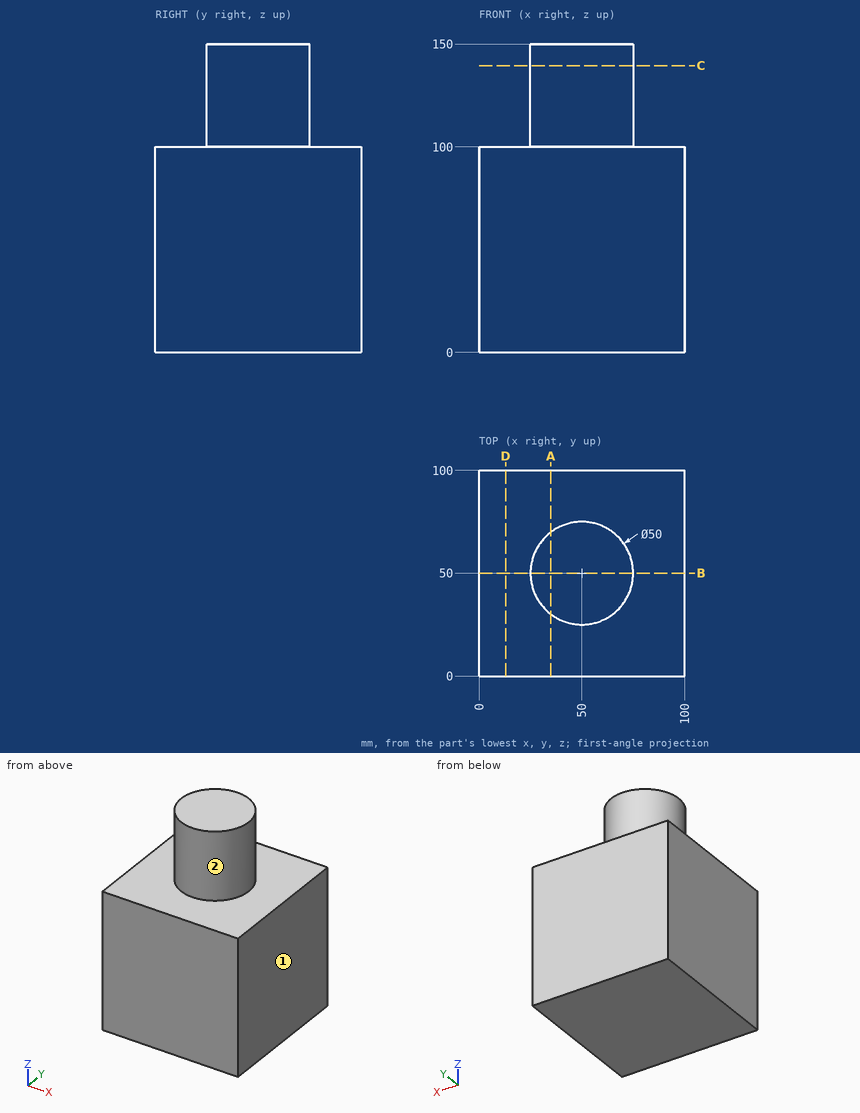
Drawing for the job (mm, zero at the part's lowest x, y, z). A direction names the side the tool comes from. Give positions to 0.01 mm unless a question says otherwise; leave off trailing zeros. Order: outer loops, then holes, each group sorted by start corner. A loop starts at its lowest first (then second) coordinate and runs counter-clockwise, first axis right, second up. Notation, with made-up numbers: M 89,-26.75 L 124,-26.75 A9 ccw 124,-19.75 Z; hole C 82,6.25 d10. An arc over 180 degrees is marked long. Write item = value, one per line. Start each with the question number.
(1) Which spindle directions (+Z, -Z, +X, -X, +Y, -Y) get a long thin tool onto all of the face, cutting with end or side? Do the marked faces 1 and 2. Say none if no direction does.
(2) Slice it at B-B on y = 50. Write the cut outline in (x, z).
(3) Slice it at A-A on x = 35. Write the cut outline in (y, z), plus the area to 3 significant figures.
(4) Slice it at D-D on x = 13. Write the cut outline in (y, z), plus the area to 3 significant figures.
(5) Pin check, flat tip, straight feed: pin 1 Ø2 at (x, y) = (87, 32.5) entering from +Z. Stop position of the tip, or through.
(6) Slice it at C-C on z = 139.5. Write the cut outline in (x, y).
(7) Probe L1, parallel to Z at x = 57, y = 87.5; L2, parallel to Y at x = 50, z = 105.5; L3, parallel to X at y = 71, z = 126. List the from-to ranges inside material, lowest first. Write a range as [from, to].
Responses:
q1.face_1 = +Z, -Z, +X, +Y, -Y
q1.face_2 = +Z
q2.outline = M 0,0 L 100,0 L 100,100 L 75,100 L 75,150 L 25,150 L 25,100 L 0,100 Z
q3.outline = M 0,0 L 100,0 L 100,100 L 70,100 L 70,150 L 30,150 L 30,100 L 0,100 Z
q3.area = 12,000 mm2
q4.outline = M 0,0 L 100,0 L 100,100 L 0,100 Z
q4.area = 10,000 mm2
q5.pin_1 = 100
q6.outline = C 50,50 d50
q7.L1 = [0, 100]
q7.L2 = [25, 75]
q7.L3 = [36.44, 63.56]
